Here's how the part is built. I have some questions about the finished solid (model axes, mm). Face numbers are marked on the shaded views. A direction names the side the tool comes from. Give positions to 0.01 mm unless a question says otherwise; leave off trailing zeros. Order: outer loops, then holes, each group sorted by start corner. A loop starts at its lowest first (then second) coordinate and runs counter-clockwise, first axis right, second up. Notation, with made-up numbers: (88.25, 12) - (98.25, 12) arc R14 cw to (98.25, 27) - close; hole circle Ø8 at (34.5, 26). An arc over 180 degrees is marked (long way). One line per question, with ' | ' between items.
from build123d import *

# Parameters (mm, degrees)
F1_DEPTH       = 39
F5_D           = 6
F5_CSINK_D     = 10
F5_CSINK_ANGLE = 90
F6_D           = 6.5
F6_CBORE_D     = 10
F6_CBORE_DEPTH = 5
F7_R           = 1
F8_SIZE        = 0.5


with BuildPart() as f1:
    # F0 (on Right) → F1 (new body)
    with BuildSketch(Plane.YZ):
        Polygon((-10, 0), (0, 0), (0, 60), (-10, 60), (-10, 42.5), (-5, 42.5), (-5, 17.5), (-10, 17.5), align=None)
    extrude(amount=F1_DEPTH)

    # F5 (through all)
    with Locations(Plane(origin=(0, 0, 0), x_dir=(-1, 0, 0), z_dir=(0, 1, 0))):
        with Locations((-29, 30), (-10, 30)):
            CounterSinkHole(F5_D / 2, F5_CSINK_D / 2, counter_sink_angle=F5_CSINK_ANGLE)

    # F6 (through all)
    with Locations(Plane.XZ.offset(10)):
        with Locations((10, 51), (29, 51), (10, 9), (29, 9)):
            CounterBoreHole(F6_D / 2, F6_CBORE_D / 2, F6_CBORE_DEPTH)

    # F7
    f7_edges = [f1.edges().sort_by_distance(p)[0] for p in [
        (39, -5, 60),
        (39, -5, 0),
        (0, -5, 60),
        (0, -5, 0),
    ]]
    fillet(f7_edges, radius=F7_R)

    # F8
    f8_edges = [f1.edges().sort_by_distance(p)[0] for p in [
        (19.5, -10, 42.5),
        (19.5, -10, 17.5),
        (39, -7.5, 42.5),
        (39, -5, 30),
        (39, -7.5, 17.5),
        (39, -10, 50.75),
        (39, -10, 9.25),
        (0, -7.5, 42.5),
        (0, -7.5, 17.5),
        (0, -10, 50.75),
        (0, 0, 30),
        (0, -5, 30),
    ]]
    chamfer(f8_edges, length=F8_SIZE)


solid = f1.part
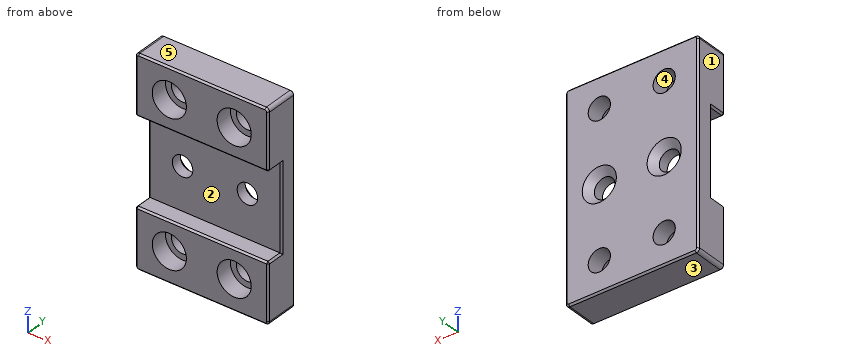
1) I want a section at B-B (y = -7.5). List the corners of the cut face in (x, z) for me, plus the area to 3 significant figures.
Model answer:
outline: (0, 1) arc R1 ccw to (1, 0) - (38, 0) arc R1 ccw to (39, 1) - (39, 17) - (38.5, 17.5) - (0.5, 17.5) - (0, 17) - close; (0, 43) - (0.5, 42.5) - (38.5, 42.5) - (39, 43) - (39, 59) arc R1 ccw to (38, 60) - (1, 60) arc R1 ccw to (0, 59) - close; hole circle Ø10 at (10, 9); hole circle Ø10 at (10, 51); hole circle Ø10 at (29, 9); hole circle Ø10 at (29, 51) | area: 1,050 mm2
2) Thinking about a two-plate mould opening in Z: for the marked faces 3, 4 and 5, which applies, +Z half, -Z half, draft (parallel to the pull), parting line (faces both ways), or undercut?
Model answer:
face 3: -Z half | face 4: undercut | face 5: +Z half
3) Please list where these lines run through material, in increasing order: L1, parallel to X at y = -2.85, z = 30; L2, parallel to Z at x = 10, y = -7.35; L3, parallel to Z at x = 10, y = -2.2.
Model answer:
L1: x = 0 to 7, 13 to 26, 32 to 39 | L2: z = 0 to 4, 14 to 17.5, 42.5 to 46, 56 to 60 | L3: z = 0 to 5.75, 12.25 to 27, 33 to 47.75, 54.25 to 60
4) I want a section at C-C (z = 30). List the corners of the cut face in (x, y) for me.
Model answer:
outline: (0, -4.5) - (0.5, -5) - (7, -5) - (7, -2) - (5, 0) - (0.5, 0) - (0, -0.5) - close; (13, -5) - (26, -5) - (26, -2) - (24, 0) - (15, 0) - (13, -2) - close; (32, -5) - (38.5, -5) - (39, -4.5) - (39, -0.5) - (38.5, 0) - (34, 0) - (32, -2) - close
5) I want a section at A-A (z = 9). List the corners of the cut face in (x, y) for me.
Model answer:
outline: (0, -9.5) - (0.5, -10) - (5, -10) - (5, -5) - (6.75, -5) - (6.75, 0) - (0.5, 0) - (0, -0.5) - close; (13.25, -5) - (15, -5) - (15, -10) - (24, -10) - (24, -5) - (25.75, -5) - (25.75, 0) - (13.25, 0) - close; (32.25, -5) - (34, -5) - (34, -10) - (38.5, -10) - (39, -9.5) - (39, -0.5) - (38.5, 0) - (32.25, 0) - close
6) On a 3-axis mill with a long thin cutter (end or side, diameter ignored), from which of +Z, -Z, +X, -X, +Y, -Y can I reach the whole of each face in a straight line? I mean the marked faces 1 and 2. Say none if no direction works.
Model answer:
face 1: +Z, -Z, -X, +Y, -Y | face 2: +X, -X, -Y
7) I'm going to push flat-ended pins straight in: P1, Ø7.5, axis at x = 29, z = 9, coming from the -Y side; P2, Ø5.5, axis at x = 10, z = 30, coming from the -Y side. Where does each tip first touch, or does it pass through?
Model answer:
P1: stops at y = -5 | P2: passes through
8) I want a section at D-D (x = 21.5). List the corners of the cut face in (y, z) for me.
Model answer:
outline: (-10, 0.5) - (-9.5, 0) - (-0.5, 0) - (0, 0.5) - (0, 59.5) - (-0.5, 60) - (-9.5, 60) - (-10, 59.5) - (-10, 43) - (-9.5, 42.5) - (-5, 42.5) - (-5, 17.5) - (-9.5, 17.5) - (-10, 17) - close
